For this review, take the finished solid that the model builds, in its own axes (mm). A direction names the side the tool comes from. Coordinates: 2 decimals unless noted, no trailing zeros. Order: outer loops, then holes, each group sorted by start corner. A loop starts at its lowest first (then second) coordinate and runs counter-clockwise, first axis right, second up.
from build123d import *

# Parameters (mm, degrees)
PIPE_TAP_DRILL_FOR_1_8_TAP1_D     = 8.4328
PIPE_TAP_DRILL_FOR_1_8_TAP1_DEPTH = 25.4
PIPE_TAP_DRILL_FOR_1_8_TAP1_TIP   = 2.533468714
CIRPATTERN1_COUNT                 = 4
SKETCH5_R                         = 6.35
BOSS_EXTRUDE1_DEPTH               = 6.35
PIPE_TAP_DRILL_FOR_1_8_TAP2_D     = 8.4328
PIPE_TAP_DRILL_FOR_1_8_TAP2_DEPTH = 6.35
PIPE_TAP_DRILL_FOR_1_8_TAP2_TIP   = 2.533468714
F_1_8_0_125_DIAMETER_HOLE4_D      = 3.175
F_1_8_0_125_DIAMETER_HOLE4_DEPTH  = 14.2875
F_10_0_1935_DIAMETER_HOLE1_D      = 4.9149
F_10_0_1935_DIAMETER_HOLE1_DEPTH  = 6.35
CIRPATTERN2_COUNT                 = 4


with BuildPart() as part:
    # Sketch1 → Revolve1 (revolve)
    with BuildSketch(Plane.XY):
        Polygon((0, 0), (-15.875, 0), (-15.875, 3.175), (-9.525, 3.175), (-9.525, 6.35), (-15.875, 6.35), (-15.875, 7.9375), (-31.75, 7.9375), (-31.75, 14.2875), (0, 14.2875), align=None)
    revolve(axis=Axis((0, 14.2875, 0), (0, -1, 0)))

    # Pipe Tap Drill for 1/8 Tap1
    with Locations(Plane.ZX.offset(14.2875)):
        with Locations((0, 0)):
            Hole(PIPE_TAP_DRILL_FOR_1_8_TAP1_D / 2, depth=PIPE_TAP_DRILL_FOR_1_8_TAP1_DEPTH)
            with Locations((0, 0, -(PIPE_TAP_DRILL_FOR_1_8_TAP1_DEPTH + PIPE_TAP_DRILL_FOR_1_8_TAP1_TIP / 2))):  # 118° drill point
                Cone(0, PIPE_TAP_DRILL_FOR_1_8_TAP1_D / 2, PIPE_TAP_DRILL_FOR_1_8_TAP1_TIP, mode=Mode.SUBTRACT)

    # Sketch3 → Cut-Revolve2 (revolve, cut)
    with BuildSketch(Plane(origin=(0, 0, 0), x_dir=(-1, 0, 0), z_dir=(0, 0, -1))):
        Polygon((-11.388289755, 5.3975), (-11.567894878, 5.217894878), (-4.900394878, -1.449605122), (-4.720789755, -1.27), align=None)
    cut_revolve2 = revolve(axis=Axis((11.567894878, 5.217894878, 0), (-0.707106781, -0.707106781, 0)), mode=Mode.SUBTRACT)

    # CirPattern1: Cut-Revolve2 ×4 about axis
    cirpattern1_axis = Axis((0, 14.2875, 0), (0, 1, 0))
    for i in range(1, CIRPATTERN1_COUNT):
        add(cut_revolve2.rotate(cirpattern1_axis, i * 360 / CIRPATTERN1_COUNT), mode=Mode.SUBTRACT)

    # Sketch5 → Boss-Extrude1 (add)
    with BuildSketch(Plane(origin=(0, 14.2875, 0), x_dir=(1, 0, 0), z_dir=(0, 1, 0))):
        with Locations((-15.24, 0)):
            Circle(SKETCH5_R)
    extrude(amount=BOSS_EXTRUDE1_DEPTH)

    # Pipe Tap Drill for 1/8 Tap2
    with Locations(Plane(origin=(-15.24, 20.6375, 0), x_dir=(0, 0, 1), z_dir=(0, 1, 0))):
        with Locations((0, 0)):
            Hole(PIPE_TAP_DRILL_FOR_1_8_TAP2_D / 2, depth=PIPE_TAP_DRILL_FOR_1_8_TAP2_DEPTH)
            with Locations((0, 0, -(PIPE_TAP_DRILL_FOR_1_8_TAP2_DEPTH + PIPE_TAP_DRILL_FOR_1_8_TAP2_TIP / 2))):  # 118° drill point
                Cone(0, PIPE_TAP_DRILL_FOR_1_8_TAP2_D / 2, PIPE_TAP_DRILL_FOR_1_8_TAP2_TIP, mode=Mode.SUBTRACT)

    # 1/8 (0.125) Diameter Hole4
    with Locations(Plane(origin=(-15.24, 20.6375, 0), x_dir=(0, 0, 1), z_dir=(0, 1, 0))):
        with Locations((0, 0)):
            Hole(F_1_8_0_125_DIAMETER_HOLE4_D / 2, depth=F_1_8_0_125_DIAMETER_HOLE4_DEPTH)

    # #10 (0.1935) Diameter Hole1
    with Locations(Plane(origin=(19.083044257, 14.2875, -19.083044257), x_dir=(0, 0, 1), z_dir=(0, 1, 0))):
        with Locations((0, 0)):
            f_10_0_1935_diameter_hole1 = Hole(F_10_0_1935_DIAMETER_HOLE1_D / 2, depth=F_10_0_1935_DIAMETER_HOLE1_DEPTH)

    # CirPattern2: #10 (0.1935) Diameter Hole1 ×4 about axis
    cirpattern2_axis = Axis((0, 0, 0), (0, 1, 0))
    for i in range(1, CIRPATTERN2_COUNT):
        add(f_10_0_1935_diameter_hole1.rotate(cirpattern2_axis, i * 360 / CIRPATTERN2_COUNT), mode=Mode.SUBTRACT)


solid = part.part
1. To check wall thickness, follow L1, parallel to Y at x = -6.5, z = -22.5; L2, parallel to Z at x = -1, y = 10.25; L3, parallel to X at y = 4, z = 3.5. State the ranges of each line that lie inside material, in increasing order.
Answer below:
L1: y = 7.94 to 14.29
L2: z = -31.73 to -4.1, 4.1 to 31.73
L3: x = -8.86 to -2.35, 2.35 to 8.86
2. The part is to be moulded in two halves that separate along Z. For faces 4 (the face through (-7, 3.175, 7)), 5 (the face through (6.883, 11.157, 30.995)), 6 (the face through (19.821, 11.068, -21.427)), say which applies: +Z half, -Z half, draft (parallel to the pull), parting line (faces both ways), or undercut.
Answer below:
face 4: draft
face 5: parting line
face 6: undercut
3. Take a section at C-C, the plane y = 17. Give the boundary of the cut face in (x, z).
Answer below:
outline: circle Ø12.7 at (-15.24, 0); hole circle Ø8.43 at (-15.24, 0)
4. Machinability: for faces 1 (the face through (-21.584, 17.418, -0.279)), 2 (the face through (7, 6.35, 7)), 3 (the face through (3.441, 1.61, 15.497)), which of the approach directions +Z, -Z, +X, -X, +Y, -Y give a long, thin tool a straight path to every point of the face, cutting with its end or side? Answer none if there is none.
Answer below:
face 1: +Y
face 2: none
face 3: -Y
5. Take a section at D-D, the plane z = 20.5. Give the boundary of the cut face in (x, y), plus the area to 3 significant figures.
Answer below:
outline: (-24.24, 7.94) - (-21.09, 7.94) - (-21.09, 14.29) - (-24.24, 14.29) - close; (-17.08, 7.94) - (17.08, 7.94) - (17.08, 14.29) - (-17.08, 14.29) - close; (21.09, 7.94) - (24.24, 7.94) - (24.24, 14.29) - (21.09, 14.29) - close
area: 257 mm2
6. Clearance check with flat-ended pins moving along their axes: pin 1 Ø5.5 at (x, z) = (-19.08, 19.08) entering from -Y; pin 2 Ø6 at (y, z) = (10, -16.5) entering from -X; pin 3 Ø3 at (y, z) = (15.5, 14) entering from +X; pin 4 Ø1.5 at (x, z) = (2, 1.5) entering from +Y. State where each tip first meets the part, or that it passes through.
Answer below:
pin 1: stops at y = 7.94
pin 2: stops at x = -28.74
pin 3: stops at x = 28.91
pin 4: passes through
